Verification items for the finished model (mm, model axes). Round coordinates to 2 decimals unless told otherwise and drop trailing zeros. Write each loop counter-clockwise with the first axis right and the second up, starting at its lowest first coordinate (ties: lowest second). Pieces come first, ordered by that corner, then holes. Notation, with made-up numbers: (37.25, 76.5) - (78.25, 76.5) arc R13 ccw to (78.25, 98.5) - close; hole circle Ø11 at (72, 53). An arc over 180 degrees is marked (long way). Answer as a JSON object with one key per item and string values. Group by question number.
1) Section check C-C (z = 0). Enter the section's corners in (x, y).
2) Section check A-A (x = 0). Enter the section's corners in (y, z), then the cut area to 3 significant figures.
3) Mould release check, pull along X, two halves, no side actions. Record for faces 1 (the flat face through (89, 3, -39)), 2 (the cylindrical face through (169.9, 1.48, -1.61)), 3 (the flat face through (-9, 2, 9)): +X half, -X half, draft (parallel to the pull), parting line (faces both ways), or undercut.
4) Thickness scan on line 1 (X direction, y = 2.4, z = 0); line 2 (Z direction, x = 175, y = 2.25); line 3 (X direction, y = 1.5, z = -2). Record the ranges inside material, lowest first.
5) Section check B-B (y = 1.5). Enter the section's corners in (x, z).
Autodesk Inventor part; units mm, degrees
ref_plane "YZ Plane" through (0, 0, 0) normal (1, 0, 0) x (0, 1, 0)
ref_plane "XZ Plane" through (0, 0, 0) normal (0, 1, 0) x (-1, 0, 0)
ref_plane "XY Plane" through (0, 0, 0) normal (0, 0, 1) x (1, 0, 0)
sketch "Sketch1" plane through (0, 0, 0) normal (0, 1, 0) x (-1, 0, 0)
  line L0 (0, 0) -> (-175, 0)
  line L1 (-175, 0) -> (-175, -80)
  line L2 (-175, -80) -> (0, -80)
  line L3 (0, -80) -> (0, 0)
  circle A0 centre (0, 0) radius 5.35
  circle A1 centre (0, -80) radius 5.35
  circle A2 centre (-175, -80) radius 5.35
  circle A3 centre (-175, 0) radius 5.35
  line L4 (12, 12) -> (-187, 12)
  line L5 (-187, 12) -> (-187, -92)
  line L6 (-187, -92) -> (12, -92)
  line L7 (12, -92) -> (12, 12)
  dimension "d0" = 175
  dimension "d1" = 80
  dimension "d2" = 10.7
  dimension "d3" = 10.7
  dimension "d4" = 10.7
  dimension "d5" = 10.7
  dimension "d6" = 12
  dimension "d7" = 12
  dimension "d8" = 12
  dimension "d9" = 12
extrude "Plate1" add sketch "Sketch1" along normal blind 3 contours L0 A0 L3 A1 L2 A2 L1 A3 | L7 L6 L5 L4
chamfer "Corner Chamfer1" distance 6 angle 45 4 edges at (-12, 1.5, 12) (187, 1.5, 12) (187, 1.5, -92) (-12, 1.5, -92)
equation "\"d3\" = d2"
equation "\"d4\" = d2"
equation "\"d5\" = d2"
equation "\"d7\" = d6"
equation "\"d8\" = d6"
equation "\"d9\" = d8"
equation "\"d10\" = Thickness"
equation "\"BendRadius\" = Thickness"
equation "\"BendReliefWidth\" = Thickness"
equation "\"BendReliefDepth\" = 0.5 * Thickness"
equation "\"CornerReliefSize\" = 4 * Thickness"
equation "\"MinimumRemnant\" = 2 * Thickness"
equation "\"TransitionRadius\" = BendRadius"
equation "\"JacobiRadiusSize\" = BendRadius"
equation "\"GapSize\" = Thickness"
properties part number "Extender" material "Stainless Steel"
Returned:
{
 "1": {"outline": "(-12, 0) - (-5.35, 0) - (-5.35, 3) - (-12, 3) - close; (5.35, 0) - (169.65, 0) - (169.65, 3) - (5.35, 3) - close; (180.35, 0) - (187, 0) - (187, 3) - (180.35, 3) - close"},
 "2": {"outline": "(0, -92) - (3, -92) - (3, -85.35) - (0, -85.35) - close; (0, -74.65) - (3, -74.65) - (3, -5.35) - (0, -5.35) - close; (0, 5.35) - (3, 5.35) - (3, 12) - (0, 12) - close", "area": "248 mm2"},
 "3": {"face 1": "draft", "face 2": "undercut", "face 3": "-X half"},
 "4": {"line 1": "-12 to -5.35, 5.35 to 169.65, 180.35 to 187", "line 2": "-92 to -85.35, -74.65 to -5.35, 5.35 to 12", "line 3": "-12 to -4.96, 4.96 to 170.04, 179.96 to 187"},
 "5": {"outline": "(-12, -86) - (-6, -92) - (181, -92) - (187, -86) - (187, 6) - (181, 12) - (-6, 12) - (-12, 6) - close; hole circle Ø10.7 at (0, -80); hole circle Ø10.7 at (0, 0); hole circle Ø10.7 at (175, -80); hole circle Ø10.7 at (175, 0)"}
}
